The model under review builds one solid part; all positions refer to its coordinate system, in mm. A direction names the side the tool comes from. Give positions to 0.01 mm unless a question says otherwise; leave off trailing zeros. Write each loop counter-clockwise with the first axis right and the second up, starting at its lowest first coordinate (ties: lowest second). Pieces come first, ordered by that corner, then holes. Notation, with made-up numbers: (-15.75, 18.25) -> (10.25, 18.25) arc R10 ccw to (10.25, 26.25) -> close; hole circle Ø4 at (4.25, -11.75). An arc over 180 degrees is marked (long way). Use CSV: the item, a comma, the result in double quotes.
```python
from build123d import *

# Parameters (mm, degrees)
CYLINDER002_R     = 0.3
CYLINDER002_DEPTH = 3
CYLINDER001_R     = 0.3
CYLINDER001_DEPTH = 3
BOX001_W          = 1
BOX001_H          = 1
BOX001_DEPTH      = 4
BOX_W             = 1
BOX_H             = 1
BOX_DEPTH         = 4
TORUS_R           = 2.2
CYLINDER_R        = 6.5
CYLINDER_DEPTH    = 21.5
FILLET_R          = 0.5


with BuildPart() as pin2:
    # Cylinder002 → Cylinder002 (new body)
    with BuildSketch(Plane(origin=(2.5, 0, -3), x_dir=(1, 0, 0), z_dir=(0, 0, 1))):
        Circle(CYLINDER002_R)
    extrude(amount=CYLINDER002_DEPTH)


with BuildPart() as pin1:
    # Cylinder001 → Cylinder001 (new body)
    with BuildSketch(Plane(origin=(-2.5, 0, -3), x_dir=(1, 0, 0), z_dir=(0, 0, 1))):
        Circle(CYLINDER001_R)
    extrude(amount=CYLINDER001_DEPTH)


with BuildPart() as box001:
    # Box001 → Box001 (new body)
    with BuildSketch(Plane(origin=(6.25, -0.5, 15), x_dir=(1, 0, 0), z_dir=(0, 0, 1))):
        with Locations((0.5, 0.5)):
            Rectangle(BOX001_W, BOX001_H)
    extrude(amount=BOX001_DEPTH)


with BuildPart() as box:
    # Box → Box (new body)
    with BuildSketch(Plane(origin=(6.25, -0.5, 7), x_dir=(1, 0, 0), z_dir=(0, 0, 1))):
        with Locations((0.5, 0.5)):
            Rectangle(BOX_W, BOX_H)
    extrude(amount=BOX_DEPTH)


with BuildPart() as ring:
    # Torus → Torus (revolve)
    with BuildSketch(Plane(origin=(0, 0, 3.5), x_dir=(1, 0, 0), z_dir=(0, -1, 0))):
        with Locations((8.2, 0)):
            Circle(TORUS_R)
    revolve(axis=Axis((0, 0, 3.5), (0, 0, 1)))


with BuildPart() as obj1:
    # Cylinder → Cylinder (new body)
    with BuildSketch(Plane.XY):
        Circle(CYLINDER_R)
    extrude(amount=CYLINDER_DEPTH)

    # Fillet
    fillet_edges = [obj1.edges().sort_by_distance(p)[0] for p in [
        (-6.5, 0, 21.5),
        (-6.5, 0, 0),
    ]]
    fillet(fillet_edges, radius=FILLET_R)

    # Cut: cut Ring
    add(ring.part, mode=Mode.SUBTRACT)

    # Cut001: cut Box
    add(box.part, mode=Mode.SUBTRACT)

    # Cut002: cut Box001
    add(box001.part, mode=Mode.SUBTRACT)

    # Fusion: union Pin1+
    add(pin1.part)

    # Fusion001: union Pin2-
    add(pin2.part)


solid = obj1.part
```
Q1. The part is to be moulded in two halves that separate along Y. For faces 1 (the flat face through (0, 0, 0)), 2 (the cylindrical face through (-5.158, -3.955, 1.291)), 3 (the flat face through (6.25, 0, 9)), say which applies: pulls with the +Y half, pulls with the -Y half, needs draft (parallel to the pull), parting line crosses it, or undercut.
Derived:
face 1,"needs draft"
face 2,"parting line crosses it"
face 3,"undercut"
Q2. Insertion check: pin 1 (0.8 mm diameter, centred on y = 0, z = 18, fed in from +X); pin 2 (6 mm diameter, centred on x = -3.5, z = 13.5, fed in from -Y); pin 3 (5 mm diameter, centred on y = -4, z = 13, fed in from -X). Each pin has a flat end and moves straight along its axis. Give the tip position at first contact, or say it passes through.
Derived:
pin 1,"stops at x = 6.25"
pin 2,"stops at y = -6.48"
pin 3,"stops at x = -6.32"
Q3. To check wall thickness, follow probe 1 along Z at (x, y) = (0.75, 3); probe 2 along Z at (x, y) = (4.25, -4.5); probe 3 along Y at (x, z) = (-3, 4). State the ranges of each line that lie inside material, in increasing order.
Derived:
probe 1,"z = 0 to 21.5"
probe 2,"z = 0.04 to 2.61, 4.39 to 21.46"
probe 3,"y = -5.26 to 5.26"
Q4. Consider section A-A (x = 0). Write out the cut boundary in (y, z), then the cut area to 3 significant figures.
Derived:
outline,"(-6.5, 0.5) arc R0.5 ccw to (-6, 0) -> (6, 0) arc R0.5 ccw to (6.5, 0.5) -> (6.5, 2.1) arc R2.2 cw to (6.5, 4.9) -> (6.5, 21) arc R0.5 ccw to (6, 21.5) -> (-6, 21.5) arc R0.5 ccw to (-6.5, 21) -> (-6.5, 4.9) arc R2.2 cw to (-6.5, 2.1) -> close"
area,"277 mm2"
Q5. Consider section C-C (z = 15.75). Write out the cut boundary in (x, y), then the cut area to 3 significant figures.
Derived:
outline,"(6.25, -0.5) -> (6.25, 0.5) -> (6.48, 0.5) arc R6.5 ccw (long way) to (6.48, -0.5) -> close"
area,"132 mm2"
Q6. Machinability: for faces 4 (the cylindrical face through (-5.158, -3.955, 12.835)), 5 (the flat face through (6.25, 0, 17)), which of the approach directions +Z, -Z, +X, -X, +Y, -Y give a long, thin tool a straight path to every point of the face, cutting with its end or side? Answer none if there is none.
Derived:
face 4,"+Z, -Z"
face 5,"+X"
Q7. Consider section B-B (y = 0). Write out the cut boundary in (x, z).
Derived:
outline,"(-6.5, 0.5) arc R0.5 ccw to (-6, 0) -> (-2.8, 0) -> (-2.8, -3) -> (-2.2, -3) -> (-2.2, 0) -> (2.2, 0) -> (2.2, -3) -> (2.8, -3) -> (2.8, 0) -> (6, 0) arc R0.5 ccw to (6.5, 0.5) -> (6.5, 2.1) arc R2.2 cw to (6.5, 4.9) -> (6.5, 7) -> (6.25, 7) -> (6.25, 11) -> (6.5, 11) -> (6.5, 15) -> (6.25, 15) -> (6.25, 19) -> (6.5, 19) -> (6.5, 21) arc R0.5 ccw to (6, 21.5) -> (-6, 21.5) arc R0.5 ccw to (-6.5, 21) -> (-6.5, 4.9) arc R2.2 cw to (-6.5, 2.1) -> close"
